The listing builds one solid part. Answer for the finished solid, in the listing's coordinates (mm). Give positions to 0.01 mm unless a question says otherwise; leave off trailing zeros. Write each loop counter-clockwise with the first axis right and the second up, starting at its lowest first coordinate (ties: lowest second). Pieces come first, ordered by that corner, then holes. Notation, with made-up numbers: (71, 8.25) - (85, 8.25) arc R20 cw to (85, 16.25) - close; hole circle Ø10 at (83.25, 14.25). An arc over 180 degrees is marked (long way). One line per question, with ' | ' between items. Start each with the question number.
1. A cutting plane is placed at C-C (y = -80). Determine the outline of the cut face in (x, z), then the cut area to 3 significant figures.
2. A cutting plane is placed at B-B (x = 240). Determine the outline of the cut face in (y, z), then the cut area to 3 significant figures.
3. Find the intervals of material crossed by L1, parallel to Y at x = 0, z = 3.1; L2, parallel to Y at x = 65, z = 4.1; L3, parallel to X at y = 20.5, z = 5.35, in increasing order. Write a range as from..to.
4. A cutting plane is placed at D-D (z = 4.5). State how many separate pieces and enclosed holes the cut face has, then the cut area to 3 significant figures.
5. Given P1, Ø9.5, axis at x = 0, y = 18, coming from the -Z side, flat-ended and moving along its own axis, determine where the tip first touches the part or whether it passes through.
6. A cutting plane is placed at A-A (y = 41.5). Determine the outline of the cut face in (x, z), then the cut area to 3 significant figures.
7. The mould has two halves that part along X. Classify faces 1 (the face through (108, 1, 0)), 2 (the face through (-18.586, 9.132, 3.972)), 3 (the face through (260, -1, 3)): +X half, -X half, draft (parallel to the pull), parting line (faces both ways), or undercut.
```python
from build123d import *

# Parameters (mm, degrees)
F0_W     = 300
F0_H     = 200
F0_R     = 4
F0_R_2   = 3
F0_R_3   = 12.5
F1_DEPTH = 6
F2_SIZE  = 3
F3_SIZE  = 2


with BuildPart() as f1:
    # F0 (on Top) → F1 (new body)
    with BuildSketch(Plane.XY):
        with Locations((110, 0)):
            Rectangle(F0_W, F0_H)
        with Locations((-20, -80)):
            Circle(F0_R, mode=Mode.SUBTRACT)
        with Locations((-15.588457, -9)):
            Circle(F0_R_2, mode=Mode.SUBTRACT)
        with Locations((0, -18)):
            Circle(F0_R_2, mode=Mode.SUBTRACT)
        with Locations((15.588457, -9)):
            Circle(F0_R_2, mode=Mode.SUBTRACT)
        with Locations((65, -19)):
            Circle(F0_R_2, mode=Mode.SUBTRACT)
        with Locations((240, -80)):
            Circle(F0_R, mode=Mode.SUBTRACT)
        with Locations((240, -41.5)):
            Circle(F0_R_2, mode=Mode.SUBTRACT)
        with Locations((-15.588457, 9)):
            Circle(F0_R_2, mode=Mode.SUBTRACT)
        Circle(F0_R_3, mode=Mode.SUBTRACT)
        with Locations((15.588457, 9)):
            Circle(F0_R_2, mode=Mode.SUBTRACT)
        with Locations((0, 18)):
            Circle(F0_R_2, mode=Mode.SUBTRACT)
        with Locations((65, 19)):
            Circle(F0_R_2, mode=Mode.SUBTRACT)
        with Locations((-20, 80)):
            Circle(F0_R, mode=Mode.SUBTRACT)
        with Locations((240, 41.5)):
            Circle(F0_R_2, mode=Mode.SUBTRACT)
        with Locations((240, 80)):
            Circle(F0_R, mode=Mode.SUBTRACT)
    extrude(amount=F1_DEPTH)

    # F2
    f2_edges = [f1.edges().sort_by_distance(p)[0] for p in [
        (-24, 80, 6),
        (236, 80, 6),
        (236, -80, 6),
        (-24, -80, 6),
    ]]
    chamfer(f2_edges, length=F2_SIZE)

    # F3
    f3_edges = [f1.edges().sort_by_distance(p)[0] for p in [
        (62, -19, 0),
        (237, -41.5, 0),
        (237, 41.5, 0),
        (62, 19, 0),
        (-3, -18, 0),
        (-18.588457, -9, 0),
        (-18.588457, 9, 0),
        (12.588457, -9, 0),
        (12.588457, 9, 0),
        (-3, 18, 0),
    ]]
    chamfer(f3_edges, length=F3_SIZE)


solid = f1.part
```
Determined:
1) outline: (-40, 0) - (-24, 0) - (-24, 3) - (-27, 6) - (-40, 6) - close; (-16, 0) - (236, 0) - (236, 3) - (233, 6) - (-13, 6) - (-16, 3) - close; (244, 0) - (260, 0) - (260, 6) - (247, 6) - (244, 3) - close | area: 1,690 mm2
2) outline: (-100, 0) - (-84, 0) - (-84, 3) - (-87, 6) - (-100, 6) - close; (-76, 0) - (-46.5, 0) - (-44.5, 2) - (-44.5, 6) - (-73, 6) - (-76, 3) - close; (-38.5, 2) - (-36.5, 0) - (36.5, 0) - (38.5, 2) - (38.5, 6) - (-38.5, 6) - close; (44.5, 2) - (46.5, 0) - (76, 0) - (76, 3) - (73, 6) - (44.5, 6) - close; (84, 0) - (100, 0) - (100, 6) - (87, 6) - (84, 3) - close | area: 1,010 mm2
3) L1: -100..-21, -15..-12.5, 12.5..15, 21..100 | L2: -100..-22, -16..16, 22..100 | L3: -40..-1.66, 1.66..62.4, 67.6..260
4) separate pieces: 1 | enclosed holes: 15 | area: 58,800 mm2
5) P1: z = 0.25
6) outline: (-40, 0) - (235, 0) - (237, 2) - (237, 6) - (-40, 6) - close; (243, 2) - (245, 0) - (260, 0) - (260, 6) - (243, 6) - close | area: 1,760 mm2
7) face 1: draft | face 2: undercut | face 3: +X half
